Autodesk Fusion 360 part; units mm, degrees
sketch "Sketch base" plane through (0, 0, 0) normal (0, 1, 0) x (1, 0, 0)
  line L0 (0, 0) -> (18, 0)
  line L1 (18, 0) -> (18, -3)
  line L2 (18, -3) -> (0, -3)
  line L3 (0, -3) -> (0, 0)
  dimension "d1" = 18
  dimension "d2" = 3
extrude "Extrude1" add sketch "Sketch base" along normal blind 38
sketch "Sketch face" plane through (0, 0, 0) normal (0, 0, -1) x (-1, 0, 0)
  line L0 (-18, 0) -> (0, 0)
  line L1 (0, 0) -> (0, 38)
  line L2 (0, 38) -> (-18, 38)
  line L3 (-18, 38) -> (-18, 0)
  circle A0 centre (-9, 35) radius 1
  circle A1 centre (-9, 6) radius 1
  line L4 (-15, 32) -> (-3, 32)
  line L5 (-3, 32) -> (-3, 9)
  line L6 (-3, 9) -> (-15, 9)
  line L7 (-15, 9) -> (-15, 32)
  line L8 (0, 0) -> (-18, 0)
  line L9 (-18, 0) -> (-18, 3)
  line L10 (-18, 3) -> (0, 3)
  line L11 (0, 3) -> (0, 0)
  dimension "d5" = 2
  dimension "d6" = 2
  dimension "d7" = 12
  dimension "d8" = 3
  dimension "d9" = 3
  dimension "d10" = 3
  dimension "d13" = 3
  dimension "d14" = 9
  dimension "d15" = 9
  dimension "d19" = 3
  dimension "d34" = 23
extrude "Extrude2" cut sketch "Sketch face" against normal blind 4 contours A0 | A1 | L4 L5 L6 L7
extrude "Extrude3" add sketch "Sketch face" along normal blind 7 and the other way blind 10 contours L0 L1 L3 L8 L9 L10 L11
hole "Hole1" at (3.5, 3, -3.5) direction (0, -1, 0) diameter 3 depth 5 tip angle 180
hole "Hole2" at (14.5, 3, 6.5) direction (0, -1, 0) diameter 3 depth 5 tip angle 180
Could you check a few things on this model? Use its own coordinates, in mm. A direction names the side the tool comes from. Round coordinates to 2 decimals unless told otherwise and drop trailing zeros. Loops run counter-clockwise (first coordinate to the right, second up) from the corner with the lowest first, then second, coordinate; pieces in that order, holes last. Notation, with made-up numbers: (-29.5, -34.5) - (9.5, -34.5) arc R24 ccw to (9.5, 4.5) - close; hole circle Ø10 at (82, -14.5). An arc over 180 degrees is marked (long way). Write item = value, one per line.
1) I'm going to push flat-ended pins straight in: P1, Ø3, axis at x = 9, y = 35, coming from the +Z side; P2, Ø8, axis at x = 3, y = 24.5, coming from the -Z side; P3, Ø7.5, axis at x = 10.5, z = -4.5, coming from the +Y side. Where does each tip first touch, or does it pass through?
Computed:
P1 = 3
P2 = 0
P3 = 3
2) Imagine slicing it at B-B (x = 11.25). Please give me the cut outline in (y, z).
Computed:
outline = (0, -7) - (3, -7) - (3, 0) - (9, 0) - (9, 3) - (3, 3) - (3, 10) - (0, 10) - close; (32, 0) - (38, 0) - (38, 3) - (32, 3) - close
3) Imagine slicing it at D-D (x = 9). Please give me the cut outline in (y, z), and give its area (3 significant figures).
Computed:
outline = (0, -7) - (3, -7) - (3, 0) - (5, 0) - (5, 3) - (3, 3) - (3, 10) - (0, 10) - close; (7, 0) - (9, 0) - (9, 3) - (7, 3) - close; (32, 0) - (34, 0) - (34, 3) - (32, 3) - close; (36, 0) - (38, 0) - (38, 3) - (36, 3) - close
area = 75.0 mm2
4) Imagine slicing it at A-A (y = 14.5). Please give me the cut outline in (x, z).
Computed:
outline = (0, 0) - (3, 0) - (3, 3) - (0, 3) - close; (15, 0) - (18, 0) - (18, 3) - (15, 3) - close
5) I need wall thicknesses on line 1 along Y through (x, z) = (9, 1.7); line 2 along X through (y, z) = (16, 1.75); line 3 along X through (y, z) = (0.9, 6.5). Which ranges of each line are inside material? Lowest first, please. Write a range as from..to.
Computed:
line_1 = 0..5, 7..9, 32..34, 36..38
line_2 = 0..3, 15..18
line_3 = 0..13, 16..18
6) On a 3-axis mill with a long thin cutter (end or side, diameter ignored), from which of +Z, -Z, +X, -X, +Y, -Y can I reach the whole of each face in a straight line? I mean faces 4 (the flat face through (3, 21, 1)), 5 (the flat face through (17, 16, 3)), 6 (the flat face through (9, 3, -3)). Say none if no direction works.
Computed:
face_4 = +Z, -Z
face_5 = +Z, +X, -X, +Y
face_6 = -Z, +X, -X, +Y
7) Imagine slicing it at C-C (z = 6.5). Please give me the cut outline in (x, y).
Computed:
outline = (0, 0) - (13, 0) - (13, 3) - (0, 3) - close; (16, 0) - (18, 0) - (18, 3) - (16, 3) - close
8) If we mould it in two halves opening along Z, with no side actions, what happens to faces 1 (the cylindrical face through (15.4, 1.5, 5.3)), 2 (the flat face through (1, 16, 0)), 3 (the flat face through (9, 32, 1))? For each: pulls with the +Z half, pulls with the -Z half, needs draft (parallel to the pull), parting line crosses it, or undercut.
Computed:
face_1 = undercut
face_2 = pulls with the -Z half
face_3 = needs draft
